```python
from build123d import *

# Parameters (mm, degrees)
SALIENTE_EXTRUIR1_DEPTH = 110
CORTAR_EXTRUIR9_DEPTH   = 55
VACIADO3_START          = 3.186974639
VACIADO3_DEPTH          = 103.813025361
VACIADO3_START_2        = 3
VACIADO3_2_DEPTH        = 0.273585229
VACIADO3_START_3        = -90
VACIADO3_3_DEPTH        = 16.944212752
CROQUIS7_R              = 9.5
CORTAR_EXTRUIR10_DEPTH  = 55


with BuildPart() as part:
    # Croquis1 → Saliente-Extruir1 (new body)
    with BuildSketch(Plane.XY):
        Polygon((0, 0), (130, 0), (130, 20), (11.547005384, 20), (-18.439456819, 71.938076074), (56.490425623, 113.447420953), (46.798692801, 130.942286341), (-45, 77.942286341), align=None)
    extrude(amount=SALIENTE_EXTRUIR1_DEPTH)

    # Croquis6 → Cortar-Extruir9 (cut, symmetric)
    with BuildSketch(Plane(origin=(-45, 77.942286341, 0), x_dir=(0.8660254037844362, 0.5000000000000044, 0), z_dir=(-0.5000000000000043, 0.866025403784436, 0))):
        with BuildLine():
            Line((51, -110.186974639), (51, -125.465118776))
            Line((51, -125.465118776), (118.324922333, -125.465118776))
            Line((118.324922333, -125.465118776), (118.324922333, 14.437296871))
            Line((118.324922333, 14.437296871), (51, 14.437296871))
            Line((51, 14.437296871), (51, -0.186974639))
            ThreePointArc((51, -0.186974639), (106, -55.186974639), (51, -110.186974639))
        make_face()
    extrude(amount=CORTAR_EXTRUIR9_DEPTH, both=True, mode=Mode.SUBTRACT)

    # Vaciado3: read off the stored shape, not the designer's step
    # Vaciado3 outline → Vaciado3 (cut)
    with BuildSketch(Plane.XY.offset(VACIADO3_START)):
        Polygon((52.412435892, 114.617890838), (44.200209183, 129.442051124), (-42.401923789, 79.442286341), (1.732050808, 3), (127, 3), (127, 17), (9.814954576, 17), (-22.564333351, 73.082571803), align=None)
    extrude(amount=VACIADO3_DEPTH, mode=Mode.SUBTRACT)

    # Vaciado3 2 outline → Vaciado3 2 (cut)
    with BuildSketch(Plane.XY.offset(VACIADO3_START_2)):
        Polygon((4.556960249, 88.107113321), (-3.430780618, 101.942286341), (-42.401923789, 79.442286341), (1.732050808, 3), (127, 3), (127, 17), (9.814954576, 17), (-22.564333351, 73.082571803), align=None)
    extrude(amount=VACIADO3_2_DEPTH, mode=Mode.SUBTRACT)

    # Vaciado3 3 outline → Vaciado3 3 (add)
    with BuildSketch(Plane(origin=(0, 0, 0), x_dir=(0.8660254037844362, 0.5000000000000042, 0), z_dir=(0.5000000000000042, -0.8660254037844363, 0)).offset(VACIADO3_START_3)):
        with BuildLine():
            ThreePointArc((68.916472868, 3.186974639), (89.973499173, 16.3789038), (103.075739879, 37.491853388))
            Line((103.075739879, 37.491853388), (103.000470437, 55.186974639))
            Line((103.000470437, 55.186974639), (102.999529567, 54.965785108))
            ThreePointArc((102.999529567, 54.965785108), (87.691266975, 18.339302693), (51, 3.186974639))
            Line((51, 3.186974639), (68.916472868, 3.186974639))
        make_face()
        with BuildLine():
            Line((103.000470437, 55.186974639), (103.075739879, 72.882095888))
            ThreePointArc((103.075739879, 72.882095888), (90.172508138, 93.794157987), (69.450214169, 107))
            Line((69.450214169, 107), (55.405723879, 107))
            ThreePointArc((55.405723879, 107), (89.220642789, 90.445767369), (102.999529567, 55.408164169))
            Line((102.999529567, 55.408164169), (103.000470437, 55.186974639))
        make_face()
        with BuildLine():
            Line((48, 3.186974639), (51, 3.186974639))
            ThreePointArc((51, 3.186974639), (49.499375014, 3.208631796), (48, 3.273585229))
            Line((48, 3.273585229), (48, 3.186974639))
        make_face()
    extrude(amount=VACIADO3_3_DEPTH)

    # Croquis7 → Cortar-Extruir10 (cut, symmetric)
    with BuildSketch(Plane(origin=(-36.277542983, 65.485784921, 0), x_dir=(0.874743269355894, 0.4845866410834722, 0), z_dir=(-0.4845866410834722, 0.874743269355894, 0))):
        with Locations(Location((49.406343615, -55.095, 0), (0, 0, 180))):
            Circle(CROQUIS7_R)
    extrude(amount=CORTAR_EXTRUIR10_DEPTH, both=True, mode=Mode.SUBTRACT)


solid = part.part
```
Input: part model. Units: mm. Frame: model coordinates. A direction names the side the tool comes from. Give positions to 0.01 mm unless a question says otherwise; leave off trailing zeros. Write each loop counter-clockwise with the first axis right and the second up, starting at its lowest first coordinate (ties: lowest second). Pieces come first, ordered by that corner, then holes. Notation, with made-up numbers: (21, 13) - (27, 13) arc R21 cw to (27, 23) - close; hole circle Ø1 at (76, -31.75). An arc over 180 degrees is marked (long way). Write item = value, one per line. Start each with the question number.
1) Cut plane D-D (x = -26). Return loops of the section in (y, z).
2) Material intervals for L1, parallel to Y at x = 111, z = 70.5; L2, parallel to Y at x = 24, z = 42; L3, parallel to Z at x = 62, y = 9.5, sorted ascending. Write a range as [from, to].
3) Cut plane B-B (y = 66.5). Return loops of the section in (x, z).
4) Cut plane C-C (z = 68). Return loops of the section in (x, y), and give its area (3 significant figures).
5) Cut plane A-A (x = 84). Return loops of the section in (y, z).
6) Draft query along Y for faces 4 (the face through (-6.15, 44.65, 54.27)), 5 (the face through (39.47, 115.33, 92.02)), 6 (the face through (-22.815, 39.517, 54.23)), 7 (the face through (29, 17, 0)). Return one class per face: pulls with the +Y half, pulls with the -Y half, needs draft (parallel to the pull), parting line crosses it, or undercut.
7) Reachability of faces 1 (the face through (-3.24, 45.61, 54.23)), 2 (the face through (127, 10, 54)), 3 (the face through (-43.514, 78.8, 55.257)) from +Z, -Z, +X, -X, +Y, -Y: full face, straight path, thin tool, end or side. Return the list, or none.
8) Pin query (flat end, axial travel): pin 1 (2 mm diameter, centred on y = 71, z = 71, fed in from -X); pin 2 (6 mm diameter, centred on x = 32.5, z = 24.5, fed in from +Y); pin 3 (5 mm diameter, centred on x = 95, z = 85.5, fed in from +Y). Return the tip coordinate at first contact, or that it passes through.
Answers follow:
q1.outline = (45.03, 0) - (88.91, 0) - (88.91, 3) - (51.03, 3) - (51.03, 107) - (88.91, 107) - (88.91, 110) - (45.03, 110) - close
q2.L1 = [0, 3], [17, 20]
q2.L2 = [0, 3], [17, 20], [95.45, 98.88]
q2.L3 = [0, 3], [107, 110]
q3.outline = (-38.39, 0) - (-15.3, 0) - (-15.3, 110) - (-38.39, 110) - close; hole (-34.93, 3) - (-18.76, 3) - (-18.76, 107) - (-34.93, 107) - close
q4.outline = (-45, 77.94) - (0, 0) - (130, 0) - (130, 20) - (11.55, 20) - (-18.44, 71.94) - (55.48, 112.89) - (45.49, 130.19) - (42.81, 128.64) - (51.27, 113.99) - (-22.56, 73.08) - (9.81, 17) - (127, 17) - (127, 3) - (1.73, 3) - (-42.4, 79.44) - close
q4.area = 1,550 mm^2
q5.outline = (0, 0) - (20, 0) - (20, 110) - (0, 110) - close; hole (3, 3) - (17, 3) - (17, 107) - (3, 107) - close
q6.face_4 = undercut
q6.face_5 = pulls with the +Y half
q6.face_6 = pulls with the -Y half
q6.face_7 = needs draft
q7.face_1 = +Z, -Z, +X
q7.face_2 = none
q7.face_3 = +Z, -Z, -X, +Y
q8.pin_1 = -41.57
q8.pin_2 = 124.42
q8.pin_3 = 20
